Can you work these out from the model? Positions are in its coordinate system, mm. A direction names the side the tool comes from. Coordinates: 2 decimals unless noted, no trailing zeros. Order: outer loops, then holes, each group sorted by start corner. A loop starts at its lowest first (then second) coordinate and runs counter-clockwise, first axis right, second up. Notation, with made-up numbers: (8, 31.5) - (48, 31.5) arc R19 cw to (48, 64.5) - close; hole circle Ø7 at (-30, 58.25). An arc over 180 degrees is marked (long way). Use a Markdown table: item, result. Add a question column.
(1) On a 3-axis mill with a long thin cutter (end or side, diameter ignored), from which of +Z, -Z, +X, -X, +Y, -Y can I reach the whole of each face in a straight line? I mean faces 1 (the cylindrical face through (-1.73, 5.97, -7.81)), 2 (the flat face through (0, 2, -24.65)), 3 (the flat face through (0, 0, -27)). Say none if no direction works.
(2) If I drill on L1, parallel to X at y = 3.5, z = -17; L2, parallel to Z at x = -16, y = 4.5; L3, parallel to Z at x = 0, y = 5, over which ranges is the centre line in solid material (lowest first)? Write a range as [from, to].
(3) I want a section at D-D (z = -7). List the corners of the cut face in (x, y) for me (3 decimals), and give its area (3 significant figures).
(4) I want a section at B-B (z = 0). List the corners of the cut face in (x, y) for me, and give its area (3 significant figures).
(5) I want a section at A-A (y = 3.25). List the corners of the cut face in (x, z) for me, and give its area (3 significant figures).
(6) For pin 1 Ø3.5 at (x, z) = (0, 0) entering from -Y; pin 2 Ø5 at (x, z) = (12.12, -7) entering from -Y; pin 3 Ø9.5 at (x, z) = (0, 0) entering from +Y, each with a flat end and sliding along its axis, tell me the tip position at first contact or that it passes through.
(7) I want a section at C-C (x = 0). List the corners of the cut face in (y, z) for me, and give its area (3 significant figures).
Autodesk Inventor part; units mm, degrees
ref_plane "YZ Plane" through (0, 0, 0) normal (1, 0, 0) x (0, 1, 0)
ref_plane "XZ Plane" through (0, 0, 0) normal (0, 1, 0) x (-1, 0, 0)
ref_plane "XY Plane" through (0, 0, 0) normal (0, 0, 1) x (1, 0, 0)
sketch "Esquisse2" plane through (0, 0, 0) normal (0, 1, 0) x (-1, 0, 0)
  line L0 (25, -30) -> (-25, -30)
  line L1 (-25, -30) -> (-25, 30)
  line L2 (-25, 30) -> (25, 30)
  line L3 (25, 30) -> (25, -30)
  point P0 (0, 0)
  dimension "d0" = 50
  dimension "d1" = 60
  dimension "d2" = 25
  dimension "d3" = 30
extrude "Extrusion1" add sketch "Esquisse2" along normal blind 11
sketch "Esquisse3" plane through (25, 0, 30) normal (1, 0, 0) x (0, 0, -1)
  line L0 (60, 0) -> (0, 0)
  line L1 (60, 0) -> (60, 11)
  line L2 (0, 0) -> (0, 11)
  circle A0 centre (7.5, 4) radius 2.15
  circle A1 centre (52.5, 4) radius 2.15
  line L3 (5.35, 4) -> (5.35, 0)
  line L4 (9.65, 4) -> (9.65, 0)
  line L5 (9.65, 0) -> (5.35, 0)
  line L6 (50.35, 4) -> (50.35, 0)
  line L7 (54.65, 4) -> (54.65, 0)
  line L8 (54.65, 0) -> (50.35, 0)
  point P0 (30, 0)
  dimension "d6" = 4.3
  dimension "d7" = 4.3
  dimension "d8" = 45
  dimension "d9" = 7.5
  dimension "d10" = 7.5
  dimension "d11" = 60
  dimension "d12" = 4
extrude "Extrusion2" cut sketch "Esquisse3" against normal through all
sketch "Esquisse4" plane through (0, 0, 0) normal (0, -1, 0) x (1, 0, 0)
  circle A0 centre (0, 0) radius 20
  dimension "d15" = 40
extrude "Extrusion3" cut sketch "Esquisse4" against normal blind 4
sketch "Esquisse5" plane through (0, 4, 0) normal (0, -1, 0) x (1, 0, 0)
  circle A0 centre (0, 0) radius 20
  circle A1 centre (0, 0) radius 8
  point P0 (8.7559, 17.9815)
  point P1 (8.7559, -17.9815)
  dimension "d18" = 16
extrude "Extrusion4" cut sketch "Esquisse5" against normal blind 4 contours A1
sketch "Esquisse7" plane through (0, 8, 0) normal (0, -1, 0) x (1, 0, 0)
  circle A0 centre (0, 0) radius 8
  circle A1 centre (0, 0) radius 3
  dimension "d24" = 6
extrude "Extrusion6" cut sketch "Esquisse7" against normal through all contours A1
sketch "Esquisse8" plane through (0, 4, 0) normal (0, -1, 0) x (1, 0, 0)
  circle A0 centre (0, 0) radius 8
  circle A1 centre (0, 14) radius 1.6
  dimension "d27" = 3.2
  dimension "d28" = 14
extrude "Extrusion7" cut sketch "Esquisse8" against normal through all contours A1
pattern_circular "Réseau circulaire1" count 3 over 360 about axis through (0, 4, 0) along (0, 1, 0) of "Extrusion7"
equation "\"d9\" = d10"
equation "\"d10\" = -0.5 * d8 + 0.5 * d11"
properties part number "Fixation_moteur" material "Plastique ABS"
Answers follow:
| question | item | result |
|---|---|---|
| 1 | face 1 | -Y |
| 1 | face 2 | +X, -X, -Y |
| 1 | face 3 | +Z, -Z, +X, -X, -Y |
| 2 | L1 | x = [-25, -10.54], [10.54, 25] |
| 2 | L2 | z = [-30, -24.59], [-20.41, 20.41], [24.59, 30] |
| 2 | L3 | z = [-30, -24.4], [-20.6, -8], [8, 12.4], [15.6, 20.6], [24.4, 30] |
| 3 | outline | (-25, 0) - (-18.735, 0) - (-18.735, 4) - (-13.724, 4) - (-13.724, 11) - (-25, 11) - close; (-10.524, 4) - (-3.873, 4) - (-3.873, 8) - (3.873, 8) - (3.873, 4) - (10.524, 4) - (10.524, 11) - (-10.524, 11) - close; (13.724, 4) - (18.735, 4) - (18.735, 0) - (25, 0) - (25, 11) - (13.724, 11) - close |
| 3 | area | 324 mm² |
| 4 | outline | (-25, 0) - (-20, 0) - (-20, 4) - (-8, 4) - (-8, 8) - (-3, 8) - (-3, 11) - (-25, 11) - close; (3, 8) - (8, 8) - (8, 4) - (20, 4) - (20, 0) - (25, 0) - (25, 11) - (3, 11) - close |
| 4 | area | 308 mm² |
| 5 | outline | (-25, -30) - (25, -30) - (25, -24.65) - (-25, -24.65) - close; (-25, -20.35) - (25, -20.35) - (25, 20.35) - (-25, 20.35) - close; (-25, 24.65) - (25, 24.65) - (25, 30) - (-25, 30) - close; hole circle Ø40 at (0, 0) |
| 5 | area | 1,310 mm² |
| 6 | pin 1 | passes through |
| 6 | pin 2 | stops at y = 4 |
| 6 | pin 3 | stops at y = 11 |
| 7 | outline | (0, -30) - (11, -30) - (11, -3) - (8, -3) - (8, -8) - (4, -8) - (4, -20) - (0, -20) - (0, -20.35) - (4, -20.35) arc R2.15 cw to (4, -24.65) - (0, -24.65) - close; (0, 20) - (4, 20) - (4, 15.6) - (11, 15.6) - (11, 30) - (0, 30) - (0, 24.65) - (4, 24.65) arc R2.15 cw to (4, 20.35) - (0, 20.35) - close; (4, 8) - (8, 8) - (8, 3) - (11, 3) - (11, 12.4) - (4, 12.4) - close |
| 7 | area | 347 mm² |
